For this review, use the dimensioned drawing (mm, ordinates from the lowest corner) and the shaded views. A direction names the side the tool comes from. Round coordinates to 2 decimals unless told otherwise and drop trailing zeros. Loops run counter-clockwise (first coordinate to the right, second up) from the corner with the lowest first, then second, coordinate; pieces in that order, holes last. Notation, with made-up numbers: (55.5, 0.5) - (110.5, 0.5) arc R17 cw to (110.5, 11.5) - close; hole circle Ø1 at (1.25, 42). An arc over 180 degrees is marked (long way). Use one line per item in the form item = value. Start each with the question number.
(1) Machinability: for the marked faces 1, 2, 3, 4 and 5, which of the approach directions +Z, -Z, +X, -X, +Y, -Y give a long, thin tool a straight path to every point of the face, cutting with its end or side? Answer none if there is none.
(2) Wall thickness on probe 1 along X at (y, z) = (37, 25.5); probe 2 along X at (y, z) = (44, 2); probe 3 along Y at (x, z) = (76, 28): over which ranges is each line inside the solid? List them lowest first. Write a range as [from, to].
(3) We need section D-D, the plane x = 63. Write out the cut boundary in (y, z), then the cut area to 3 significant figures.
(4) We need section B-B, the plane z = 43. Write out the cut boundary in (x, y), then the cut area to 3 significant figures.
(5) The part is to be moulded in two halves that separate along X. For the marked faces 6, 7 and 8, say which applies: released by +X, released by -X, zero draft, split by the parting line, or undercut.
(6) We need section A-A, the plane y = 36.5. Write out the cut boundary in (x, z), then the cut area to 3 significant figures.
(7) For pin 1 (24 mm diameter, centred on y = 36, z = 38, fed in from +X); pin 2 (16 mm diameter, centred on y = 33.5, z = 13.5, fed in from +X); pin 3 (15 mm diameter, centred on y = 28, z = 37, fed in from -X); pin 4 (10 mm diameter, centred on x = 46.5, z = 26, fed in from +Y), all flat-tipped, find the tip position at first contact; note any pin that passes through.
(8) We need section C-C, the plane y = 26. Write out the cut boundary in (x, z).
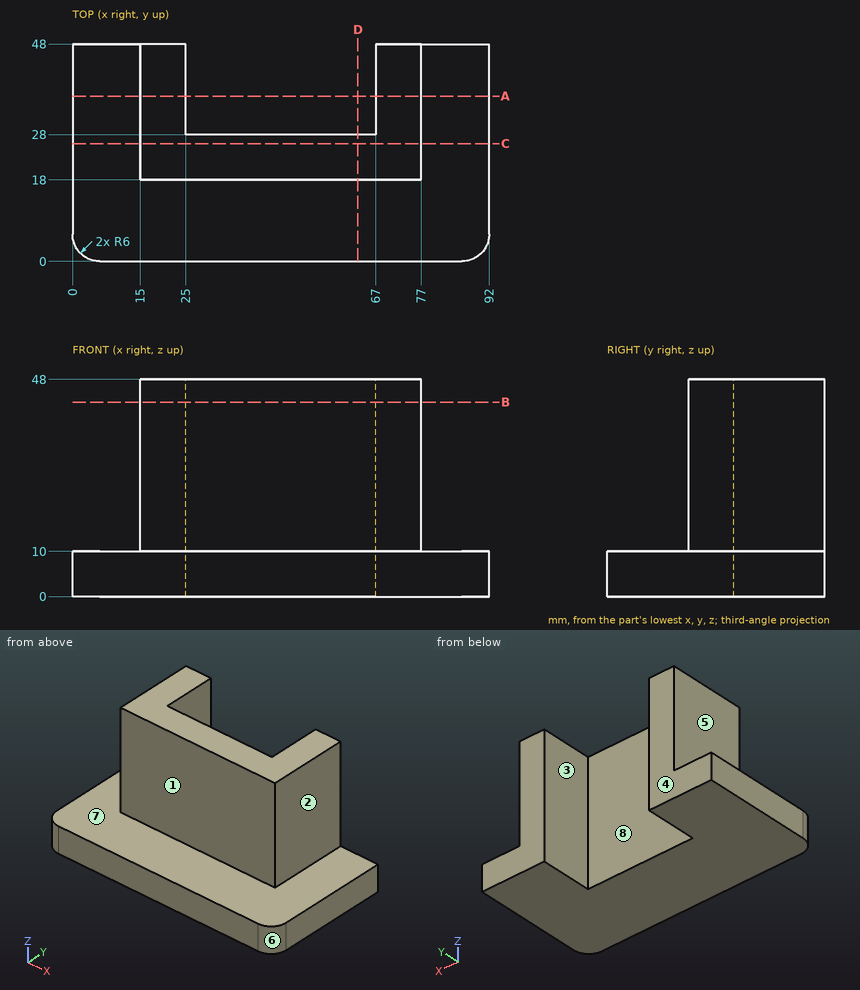
Data:
q1.face_1 = +Z, +X, -X, -Y
q1.face_2 = +Z, +X, +Y, -Y
q1.face_3 = +Z, -Z, +Y
q1.face_4 = +Z, -Z, +X, -X, +Y
q1.face_5 = +Z, -X, +Y, -Y
q2.probe_1 = [15, 25], [67, 77]
q2.probe_2 = [0, 25], [67, 92]
q2.probe_3 = [18, 48]
q3.outline = (0, 0) - (28, 0) - (28, 48) - (18, 48) - (18, 10) - (0, 10) - close
q3.area = 660 mm^2
q4.outline = (15, 18) - (77, 18) - (77, 48) - (67, 48) - (67, 28) - (25, 28) - (25, 48) - (15, 48) - close
q4.area = 1,020 mm^2
q5.face_6 = released by +X
q5.face_7 = zero draft
q5.face_8 = undercut
q6.outline = (0, 0) - (25, 0) - (25, 48) - (15, 48) - (15, 10) - (0, 10) - close; (67, 0) - (92, 0) - (92, 10) - (77, 10) - (77, 48) - (67, 48) - close
q6.area = 1,260 mm^2
q7.pin_1 = 77
q7.pin_2 = 92
q7.pin_3 = 15
q7.pin_4 = 28
q8.outline = (0, 0) - (92, 0) - (92, 10) - (77, 10) - (77, 48) - (15, 48) - (15, 10) - (0, 10) - close
